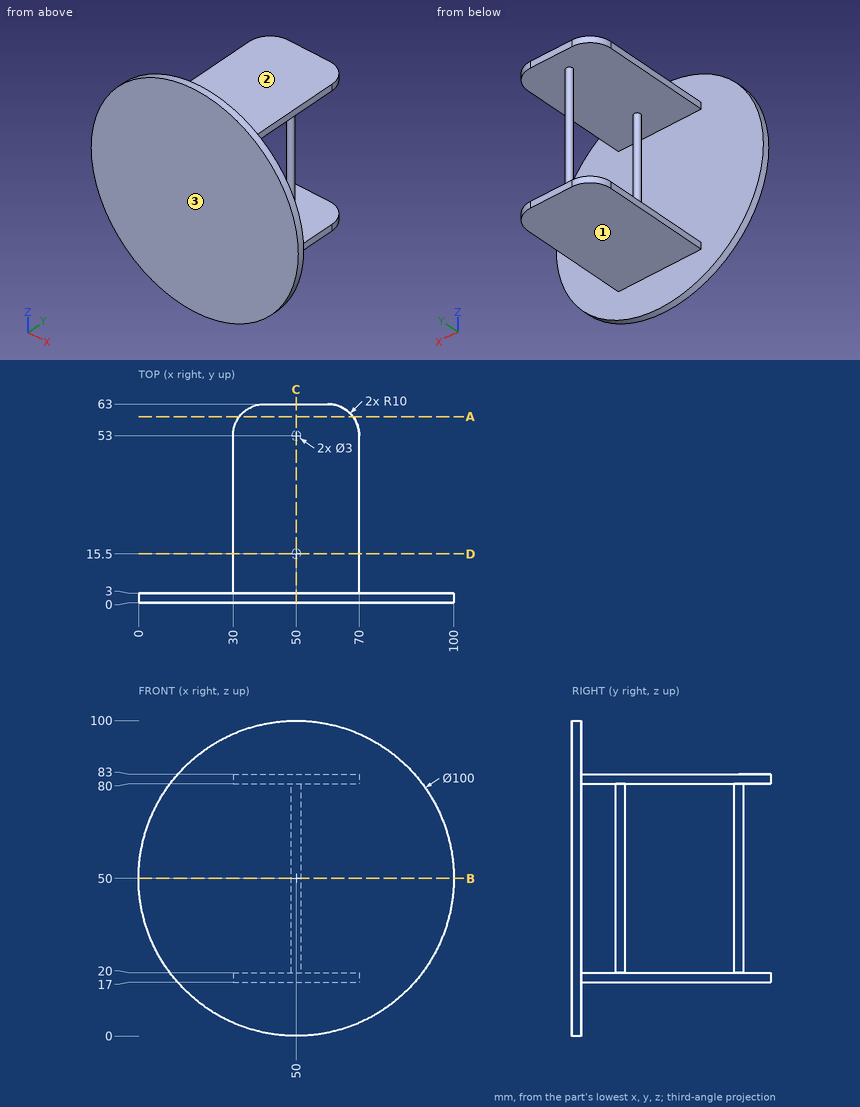
Drawing for the job (mm, zero at the part's lowest x, y, z). A direction names the side the tool comes from. Round coordinates to 2 decimals unless told otherwise and drop trailing zeros. Loops run counter-clockwise (first coordinate to the right, second up) from the corner with the lowest first, then second, coordinate; pieces in that order, holes last. Notation, with made-up numbers: M 23,38.5 L 47,38.5 A16 cw 47,64.5 Z; hole C -13.75,6.25 d2. An arc over 180 degrees is marked long. Use a Markdown table: item, result. Add a question column.
(1) Cut at D-D (y = 15.5). Give the cut face in (x, z).
(2) Which spindle directions (+Z, -Z, +X, -X, +Y, -Y) get a long thin tool onto all of the face, cutting with end or side? Do the marked faces 1, 2 and 3. Say none if no direction does.
(3) Cut at A-A (y = 59). Give the cut face in (x, z).
(4) Flat gauge pins, fed straight in: pin 1 (3.5 mm diameter, centred on y = 32.5, z = 81.5, fed in from -X); pin 2 (1.5 mm diameter, centred on x = 69.5, y = 6.5, fed in from +Z); pin 3 (12 mm diameter, centred on x = 89, z = 19.5, fed in from +Y); pin 4 (10 mm diameter, centred on x = 21.5, y = 21.5, fed in from -Z). Where does each tip first touch, or does it go through?
(5) Cut at C-C (x = 50). Give the cut face in (y, z).
(6) Cut at B-B (z = 50). Give the cut face in (x, y).
(7) Drill centre lines: line 1 (Z direction, x = 61, y = 60); line 2 (Y direction, x = 20, z = 65); line 3 (Y direction, x = 50.5, z = 76). Where is each one in solid material? Low to high.
Geometry says:
| question | item | result |
|---|---|---|
| 1 | outline | M 30,17 L 70,17 L 70,20 L 51.5,20 L 51.5,80 L 70,80 L 70,83 L 30,83 L 30,80 L 48.5,80 L 48.5,20 L 30,20 Z |
| 2 | face 1 | -Z, +X, -X, +Y |
| 2 | face 2 | +Z, +X, -X, +Y |
| 2 | face 3 | +Z, -Z, +X, -X, -Y |
| 3 | outline | M 32,17 L 68,17 L 68,20 L 32,20 Z; M 32,80 L 68,80 L 68,83 L 32,83 Z |
| 4 | pin 1 | stops at x = 30 |
| 4 | pin 2 | stops at z = 83 |
| 4 | pin 3 | stops at y = 3 |
| 4 | pin 4 | passes through |
| 5 | outline | M 0,0 L 3,0 L 3,17 L 63,17 L 63,20 L 54.5,20 L 54.5,80 L 63,80 L 63,83 L 3,83 L 3,100 L 0,100 Z; hole M 3,20 L 14,20 L 14,80 L 3,80 Z; hole M 17,20 L 51.5,20 L 51.5,80 L 17,80 Z |
| 6 | outline | M 0,0 L 100,0 L 100,3 L 0,3 Z; C 50,15.5 d3; C 50,53 d3 |
| 7 | line 1 | z = 17 to 20, 80 to 83 |
| 7 | line 2 | y = 0 to 3 |
| 7 | line 3 | y = 0 to 3, 14.09 to 16.91, 51.59 to 54.41 |
